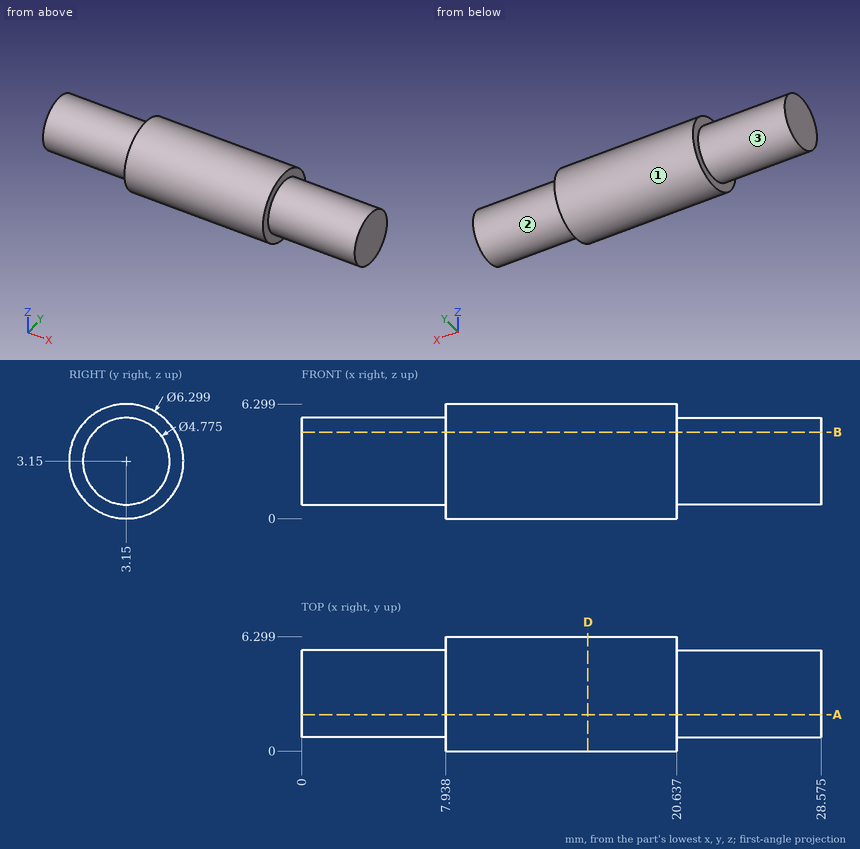
The figure shows three views and two pictorial views of one solid part (mm, origin at its lowest corner). Answer the questions. A direction names the side the tool comes from. Coordinates: 2 decimals unless noted, no trailing zeros. Loops run counter-clockwise (first coordinate to the right, second up) from the corner with the lowest first, then second, coordinate; pieces in that order, holes last. Notation, with made-up numbers: (-35.5, 40.5) - (-26.5, 40.5) arc R10 ccw to (-26.5, 53.5) - close; hole circle Ø2 at (73.5, 51). An arc over 180 degrees is marked (long way). Answer in a Markdown table with one row per item.
Q1. For the marked faces 1, 2 and 3, determine the directions among +Z, -Z, +X, -X, +Y, -Y from which every point of the face is accessible in a straight line to the end or side of a thin tool.
Here are the results:
| item | result |
|---|---|
| face 1 | +X, -X |
| face 2 | +X |
| face 3 | -X |
Q2. Find section B-B on z = 4.75. Write down the section's boundary in (x, y) (1 decimal), plus the area to 3 significant figures.
Here are the results:
| item | result |
|---|---|
| outline | (0, 1.4) - (7.9, 1.4) - (7.9, 0.4) - (20.6, 0.4) - (20.6, 1.4) - (28.6, 1.4) - (28.6, 4.9) - (20.6, 4.9) - (20.6, 5.9) - (7.9, 5.9) - (7.9, 4.9) - (0, 4.9) - close |
| area | 125 mm^2 |
Q3. Find section D-D on x = 15.75. Write down the section's boundary in (y, z).
Here are the results:
| item | result |
|---|---|
| outline | circle Ø6.3 at (3.15, 3.15) |
Q4. Straight lines are drawn through the part: line 1 along X through (y, z) = (3.25, 0.5); line 2 along Z through (x, y) = (22.5, 3); line 3 along Y through (x, z) = (13.5, 6) (1 decimal). For each, find the intervals that lie inside material, in ascending order. Write a range as [from, to].
Here are the results:
| item | result |
|---|---|
| line 1 | x = [7.94, 20.64] |
| line 2 | z = [0.77, 5.53] |
| line 3 | y = [1.8, 4.5] |
Q5. Find section A-A on y = 2. Write down the section's boundary in (x, z) (1 decimal), plus the area to 3 significant figures.
Here are the results:
| item | result |
|---|---|
| outline | (0, 1.1) - (7.9, 1.1) - (7.9, 0.2) - (20.6, 0.2) - (20.6, 1.1) - (28.6, 1.1) - (28.6, 5.2) - (20.6, 5.2) - (20.6, 6.1) - (7.9, 6.1) - (7.9, 5.2) - (0, 5.2) - close |
| area | 141 mm^2 |
Q6. Given P1, Ø1, axis at x = 14, y = 5.5, coming from the -Z side, flat-ended and moving along its own axis, determine where the tip first touches the part or whether it passes through.
Here are the results:
| item | result |
|---|---|
| P1 | stops at z = 0.6 |
